```python
from build123d import *

# Parameters (mm, degrees)
SKETCH1_W           = 45
SKETCH1_H           = 60
BOSS_EXTRUDE1_DEPTH = 15
SKETCH2_R           = 4.05
SKETCH2_W           = 10
SKETCH2_H           = 25
CUT_EXTRUDE1_DEPTH  = 46
SKETCH3_W           = 17
SKETCH3_H           = 12
BOSS_EXTRUDE2_DEPTH = 45
SKETCH4_W           = 25
SKETCH4_H           = 17
BOSS_EXTRUDE3_DEPTH = 18
SKETCH5_W           = 2
SKETCH5_H           = 30
CUT_EXTRUDE2_DEPTH  = 5
SKETCH6_R           = 4.5
CUT_EXTRUDE3_DEPTH  = 61
SKETCH7_R           = 7.5
SKETCH7_R_2         = 5
SKETCH7_R_3         = 1.25
CUT_EXTRUDE4_DEPTH  = 27
SKETCH8_R           = 15
SKETCH8_R_2         = 1.5
CUT_EXTRUDE5_DEPTH  = 22
FILLET1_R           = 6
SKETCH9_R           = 1.5
CUT_EXTRUDE6_DEPTH  = 15
SKETCH10_R          = 1.5
CUT_EXTRUDE7_DEPTH  = 5
CUT_EXTRUDE8_START  = -60
SKETCH10_2_R        = 1.5
CUT_EXTRUDE8_DEPTH  = 5


with BuildPart() as part:
    # Sketch1 → Boss-Extrude1 (new body)
    with BuildSketch(Plane.XY):
        Rectangle(SKETCH1_W, SKETCH1_H)
    extrude(amount=BOSS_EXTRUDE1_DEPTH)

    # Sketch2 → Cut-Extrude1 (cut, through all)
    with BuildSketch(Plane(origin=(22.5, 0, 0), x_dir=(0, 0, -1), z_dir=(1, 0, 0))):
        with Locations((-7.5, 22.5)):
            Circle(SKETCH2_R)
        with Locations((-7.5, -22.5)):
            Circle(SKETCH2_R)
        with Locations((-7.5, 0)):
            Rectangle(SKETCH2_W, SKETCH2_H)
    extrude(amount=-CUT_EXTRUDE1_DEPTH, mode=Mode.SUBTRACT)

    # Sketch3 → Boss-Extrude2 (add)
    with BuildSketch(Plane.ZY.offset(22.5)):
        with Locations((23.5, -24)):
            Rectangle(SKETCH3_W, SKETCH3_H)
    extrude(amount=-BOSS_EXTRUDE2_DEPTH)

    # Sketch4 → Boss-Extrude3 (add)
    with BuildSketch(Plane(origin=(0, -18, 0), x_dir=(1, 0, 0), z_dir=(0, 1, 0))):
        with Locations((10, -23.5)):
            Rectangle(SKETCH4_W, SKETCH4_H)
    extrude(amount=BOSS_EXTRUDE3_DEPTH)

    # Sketch5 → Cut-Extrude2 (cut)
    with BuildSketch(Plane.XY.offset(32)):
        with Locations((10, -15)):
            Rectangle(SKETCH5_W, SKETCH5_H)
    extrude(amount=-CUT_EXTRUDE2_DEPTH, mode=Mode.SUBTRACT)

    # Sketch6 → Cut-Extrude3 (cut, through all)
    with BuildSketch(Plane.XZ.offset(30)):
        with Locations((10, 23)):
            Circle(SKETCH6_R)
    extrude(amount=-CUT_EXTRUDE3_DEPTH, mode=Mode.SUBTRACT)

    # Sketch7 → Cut-Extrude4 (cut)
    with BuildSketch(Plane.XZ.offset(30)):
        with Locations((10, 23)):
            Circle(SKETCH7_R)
        with Locations((-11.1, 23)):
            Circle(SKETCH7_R_2)
        with Locations((-3.6, 23)):
            Circle(SKETCH7_R_3)
        with Locations((-11.1, 30.5)):
            Circle(SKETCH7_R_3)
        with Locations((-11.1, 15.5)):
            Circle(SKETCH7_R_3)
        with Locations((-18.6, 23)):
            Circle(SKETCH7_R_3)
    extrude(amount=-CUT_EXTRUDE4_DEPTH, mode=Mode.SUBTRACT)

    # Sketch8 → Cut-Extrude5 (cut)
    with BuildSketch(Plane(origin=(0, 0, 0), x_dir=(-1, 0, 0), z_dir=(0, 0, -1))):
        with Locations((2.5, 0)):
            Circle(SKETCH8_R)
        with Locations((18.25, 15.75)):
            Circle(SKETCH8_R_2)
        with Locations((-13.25, 15.75)):
            Circle(SKETCH8_R_2)
        with Locations((-13.25, -15.75)):
            Circle(SKETCH8_R_2)
        with Locations((18.25, -15.75)):
            Circle(SKETCH8_R_2)
    extrude(amount=-CUT_EXTRUDE5_DEPTH, mode=Mode.SUBTRACT)

    # Fillet1
    fillet1_edges = [part.edges().sort_by_distance(p)[0] for p in [
        (-22.5, -24, 32),
        (-2.5, -9, 32),
        (22.5, -15, 32),
    ]]
    fillet(fillet1_edges, radius=FILLET1_R)

    # Sketch9 → Cut-Extrude6 (cut)
    with BuildSketch(Plane(origin=(0, 0, 0), x_dir=(-1, 0, 0), z_dir=(0, 0, -1))):
        with Locations((-18, 0)):
            Circle(SKETCH9_R)
    extrude(amount=-CUT_EXTRUDE6_DEPTH, mode=Mode.SUBTRACT)

    # Sketch10 → Cut-Extrude7 (cut)
    with BuildSketch(Plane(origin=(0, 30, 0), x_dir=(1, 0, 0), z_dir=(0, 1, 0))):
        with Locations((-15, -7.5)):
            Circle(SKETCH10_R)
        with Locations((15, -7.5)):
            Circle(SKETCH10_R)
    extrude(amount=-CUT_EXTRUDE7_DEPTH, mode=Mode.SUBTRACT)

    # Sketch10<2> → Cut-Extrude8 (cut)
    with BuildSketch(Plane(origin=(0, 30, 0), x_dir=(1, 0, 0), z_dir=(0, 1, 0)).offset(CUT_EXTRUDE8_START)):
        with Locations((-15, -7.5)):
            Circle(SKETCH10_2_R)
        with Locations((15, -7.5)):
            Circle(SKETCH10_2_R)
    extrude(amount=CUT_EXTRUDE8_DEPTH, mode=Mode.SUBTRACT)


solid = part.part
```
Part model, mm, in its own coordinate system. A direction names the side the tool comes from. Round coordinates to 2 decimals unless told otherwise and drop trailing zeros. Order: outer loops, then holes, each group sorted by start corner. A loop starts at its lowest first (then second) coordinate and runs counter-clockwise, first axis right, second up. Notation, with made-up numbers: M 31.25,40.5 L 47.25,40.5 A20 ccw 47.25,55.5 Z; hole C 73.5,2 d9. An arc over 180 degrees is marked long. Answer in a Markdown table with one row per item. Add a question column.
Q1. Cut at A-A on y = 22.5. Give the cut face in (x, z).
Q2. Pin check, flat tips, straight feed: pin 1 (13.5 mm diameter, centred on x = 4.5, y = 11.5, fed in from +Z); pin 2 (5 mm diameter, centred on x = -6, z = 27, fed in from +Y); pin 3 (7.5 mm diameter, centred on y = -22.5, z = 7.5, fed in from -X); pin 4 (2.5 mm diameter, centred on x = -15, z = 7.5, fed in from -Y). Stop position of each tip, or through.
Q3. Cut at B-B on x = -18.6. Give the cut face in (y, z).
Q4. Mould opens along X. For faces 1 (the face through (20.789, -14.79, 30.196)), 2 (the face through (6, -3, 26)), 3 (the face through (0.315, 18.546, 8.378)) say: +X half, -X half, draft (parallel to the pull), parting line (faces both ways), or undercut.
Q5. Cut at C-C on y = -22.5. Give the cut face in (x, z).
Q6. Wall check: L1, parallel to X at y = 0, z = 13.25; L2, parallel to X at y = -10, z = 23; L3, parallel to X at y = -2, z = 23. Give the ranges that are in metal, low to high. Write a range as from..to.
Q7. 3-axis set-ups, long thin cutter, end or side, ignore diameter. For faces 4 (the face through (-19, 0, 2.5)), 5 (the face through (13.5, 28.16, 7.43)), 6 (the face through (-0.789, -8.874, 30.196)): which of +Z, -Z, +X, -X, +Y, -Y reach the whole face in a straight line?
Q8. Cut at D-D on x = 1. Give the cut face in (y, z).
Established:
| question | item | result |
|---|---|---|
| 1 | outline | M -22.5,0 L 22.5,0 L 22.5,3.45 L -22.5,3.45 Z; M -22.5,11.55 L 22.5,11.55 L 22.5,15 L -22.5,15 Z |
| 2 | pin 1 | stops at z = 15 |
| 2 | pin 2 | stops at y = -18 |
| 2 | pin 3 | passes through |
| 2 | pin 4 | stops at y = -18.65 |
| 3 | outline | M -30,0 L -17.21,0 L -17.21,15 L -18,15 L -18,21.75 L -30,21.75 Z; M -30,24.25 L -18,24.25 L -18,31.62 L -30,31.62 Z; M -14.29,0 L 14.29,0 L 14.29,15 L -14.29,15 Z; M 17.21,0 L 30,0 L 30,15 L 17.21,15 Z; hole C -22.5,7.5 d8.1; hole M -12.5,2.5 L 12.5,2.5 L 12.5,12.5 L -12.5,12.5 Z; hole C 22.5,7.5 d8.1 |
| 4 | face 1 | +X half |
| 4 | face 2 | undercut |
| 4 | face 3 | draft |
| 5 | outline | M -22.5,0 L 22.5,0 L 22.5,3.45 L -22.5,3.45 Z; M -22.5,11.55 L 22.5,11.55 L 22.5,26 A6 ccw 16.5,32 L 11,32 L 11,30.43 A7.5 cw long 9,30.43 L 9,32 L -16.5,32 A6 ccw -22.5,26 Z; hole C -18.6,23 d2.5; hole C -11.1,23 d10; hole C -11.1,15.5 d2.5; hole C -11.1,30.5 d2.5; hole C -3.6,23 d2.5 |
| 6 | L1 | x = -22.5..-17.5, 12.5..16.5, 19.5..22.5 |
| 6 | L2 | x = -2.35..2.5, 17.5..22.5 |
| 6 | L3 | x = -2.5..5.5, 14.5..22.5 |
| 7 | face 4 | +X, -X |
| 7 | face 5 | +Y |
| 7 | face 6 | +Z, -X, +Y |
| 8 | outline | M -30,0 L -14.59,0 L -14.59,22 L 0,22 L 0,31.45 L -18,31.45 L -18,32 L -30,32 Z; M 14.59,0 L 30,0 L 30,15 L 14.59,15 Z; hole C -22.5,7.5 d8.1; hole C 22.5,7.5 d8.1 |
